Part model, mm, in its own coordinate system. A direction names the side the tool comes from. Coordinates: 2 decimals unless noted, no trailing zeros. Write each loop counter-clockwise with the first axis right and the second up, starting at its lowest first coordinate (ties: lowest second). Pieces come first, ordered by that corner, then holes. Notation, with made-up numbers: (37, 42.5) - (60, 42.5) arc R32 cw to (60, 71.5) - close; hole circle Ø4 at (88.25, -21.5). An arc over 180 degrees is marked (long way). Use a Markdown table: item, result.
```python
from build123d import *

# Parameters (mm, degrees)
ESQUISSE1_W             = 40
ESQUISSE1_H             = 60
ESQUISSE1_R             = 2.6
BOSS_EXTRU_1_DEPTH      = 5
ESQUISSE2_W             = 23.1
ESQUISSE2_H             = 14
ENL_V_MAT_EXTRU_1_DEPTH = 73.284161474
CONG_1_R                = 2
CONG_2_R                = 0.4
ESQUISSE3_R             = 1
ENL_V_MAT_EXTRU_2_DEPTH = 73.284161474
ESQUISSE4_W             = 48.028106485
ESQUISSE4_H             = 39.571936154
ENL_V_MAT_EXTRU_3_DEPTH = 10
CONG_3_R                = 2


with BuildPart() as part:
    # Esquisse1 → Boss.-Extru.1 (new body)
    with BuildSketch(Plane.XY):
        with Locations((20, 30)):
            Rectangle(ESQUISSE1_W, ESQUISSE1_H)
        with Locations((5, 30)):
            Circle(ESQUISSE1_R, mode=Mode.SUBTRACT)
        with Locations((35, 30)):
            Circle(ESQUISSE1_R, mode=Mode.SUBTRACT)
    extrude(amount=BOSS_EXTRU_1_DEPTH)

    # Esquisse2 → Enlèv. mat.-Extru.1 (cut, through all)
    with BuildSketch(Plane.XY.offset(5)):
        with BuildLine():
            Line((5, 27.4), (0, 27.4))
            ThreePointArc((0, 27.4), (-2.6, 30), (0, 32.6))
            Line((0, 32.6), (5, 32.6))
            ThreePointArc((5, 32.6), (7.6, 30), (5, 27.4))
        make_face()
        with BuildLine():
            Line((35, 32.6), (40, 32.6))
            ThreePointArc((40, 32.6), (42.6, 30), (40, 27.4))
            Line((40, 27.4), (35, 27.4))
            ThreePointArc((35, 27.4), (32.4, 30), (35, 32.6))
        make_face()
        with Locations((20, 53)):
            Rectangle(ESQUISSE2_W, ESQUISSE2_H)
        with Locations((20, 7)):
            Rectangle(ESQUISSE2_W, ESQUISSE2_H)
    extrude(amount=-ENL_V_MAT_EXTRU_1_DEPTH, mode=Mode.SUBTRACT)

    # Congé1
    cong_1_edges = [part.edges().sort_by_distance(p)[0] for p in [
        (0, 27.4, 2.5),
        (0, 32.6, 2.5),
        (40, 32.6, 2.5),
        (40, 27.4, 2.5),
        (8.45, 60, 2.5),
        (31.55, 60, 2.5),
        (8.45, 0, 2.5),
        (31.55, 0, 2.5),
        (0, 60, 2.5),
        (40, 60, 2.5),
        (40, 0, 2.5),
        (0, 0, 2.5),
    ]]
    fillet(cong_1_edges, radius=CONG_1_R)

    # Congé2
    cong_2_edges = [part.edges().sort_by_distance(p)[0] for p in [
        (8.45, 46, 2.5),
        (31.55, 46, 2.5),
        (8.45, 14, 2.5),
        (31.55, 14, 2.5),
    ]]
    fillet(cong_2_edges, radius=CONG_2_R)

    # Esquisse3 → Enlèv. mat.-Extru.2 (cut, through all)
    with BuildSketch(Plane.XY.offset(5)):
        with Locations((34, 52.5)):
            Circle(ESQUISSE3_R)
        with Locations((6, 52.5)):
            Circle(ESQUISSE3_R)
        with Locations(Location((6, 7.5, 0), (0, 0, 180))):
            Circle(ESQUISSE3_R)
        with Locations(Location((34, 7.5, 0), (0, 0, 180))):
            Circle(ESQUISSE3_R)
    extrude(amount=-ENL_V_MAT_EXTRU_2_DEPTH, mode=Mode.SUBTRACT)

    # Esquisse4 → Enlèv. mat.-Extru.3 (cut)
    with BuildSketch(Plane.XY.offset(5)):
        with Locations((15.985946757, -4.785968077)):
            Rectangle(ESQUISSE4_W, ESQUISSE4_H)
    extrude(amount=-ENL_V_MAT_EXTRU_3_DEPTH, mode=Mode.SUBTRACT)

    # Congé3
    cong_3_edges = [part.edges().sort_by_distance(p)[0] for p in [
        (0, 15, 2.5),
        (40, 15, 2.5),
    ]]
    fillet(cong_3_edges, radius=CONG_3_R)


solid = part.part
```
Item 1: Two-plate mould, pull along X, no slides. Class faces 5 (the face through (0.6, 59.43, 2.54)), 6 (the face through (39.43, 59.4, 2.54)), 7 (the face through (32.15, 59.43, 2.46)), 8 (the face through (20, 33, 5)): pulls with the +X half, pulls with the -X half, needs draft (parallel to the pull), parting line crosses it, or undercut.
From the geometry:
| item | result |
|---|---|
| face 5 | pulls with the -X half |
| face 6 | pulls with the +X half |
| face 7 | undercut |
| face 8 | needs draft |
Item 2: Band-saw the part on A-A, the plane y = 49. Give the cut face in (x, z).
From the geometry:
| item | result |
|---|---|
| outline | (0, 0) - (8.45, 0) - (8.45, 5) - (0, 5) - close; (31.55, 0) - (40, 0) - (40, 5) - (31.55, 5) - close |
Item 3: Drill centre lines: probe 1 along X at (y, z) = (48, 4.7); probe 2 along Y at (x, z) = (6, 1.15); probe 3 along Y at (x, z) = (35.5, 2.85). Where is each one in solid material? Low to high.
From the geometry:
| item | result |
|---|---|
| probe 1 | 0 to 8.45, 31.55 to 40 |
| probe 2 | 15 to 27.6, 32.4 to 51.5, 53.5 to 60 |
| probe 3 | 15 to 27.4, 32.6 to 60 |
Item 4: Band-saw the part on C-C, the plane y = 30. Give the cut face in (x, z), then the cut area to 3 significant figures.
From the geometry:
| item | result |
|---|---|
| outline | (7.6, 0) - (32.4, 0) - (32.4, 5) - (7.6, 5) - close |
| area | 124 mm^2 |
Item 5: Band-saw the part on B-B, the plane z = 2.2. Count the separate pieces of the cut face and the enclosed holes in it, then the cut area to 3 significant figures.
From the geometry:
| item | result |
|---|---|
| separate pieces | 1 |
| enclosed holes | 2 |
| area | 1,390 mm^2 |
Item 6: Which spindle directions (+Z, -Z, +X, -X, +Y, -Y) get a long thin tool onto all of the face, cutting with end or side? Do faces 1 (the face through (20, 33, 0)), 2 (the face through (37, 27.4, 3)), 3 (the face through (31.55, 52, 3)), 4 (the face through (0.57, 33.2, 2.46)). Say none if no direction does.
From the geometry:
| item | result |
|---|---|
| face 1 | -Z, +X, -X, +Y, -Y |
| face 2 | +Z, -Z, +X |
| face 3 | +Z, -Z, +Y |
| face 4 | +Z, -Z, -X |
Item 7: Band-saw the part on D-D, the plane x = 11.5. Give the cut face in (y, z), then the cut area to 3 significant figures.
From the geometry:
| item | result |
|---|---|
| outline | (15, 0) - (46, 0) - (46, 5) - (15, 5) - close |
| area | 155 mm^2 |
Item 8: Drop flat-ended pins along their axis: P1, Ø5, axis at x = 22, y = 23.5, coming from the -Z side; P2, Ø1.8, axis at x = 6, y = 52.5, coming from the +Z side; P3, Ø2, axis at y = 31, z = 2.5, coming from the +X side. Give the stop position or say it passes through.
From the geometry:
| item | result |
|---|---|
| P1 | z = 0 |
| P2 | through |
| P3 | x = 33.34 |
